CAD build for the part. Positions are in the model's coordinates, mm. A direction names the side the tool comes from. Round coordinates to 2 decimals unless told otherwise and drop trailing zeros. Loops run counter-clockwise (first coordinate to the right, second up) from the corner with the lowest first, then second, coordinate; pieces in that order, holes last. Notation, with made-up numbers: (-35.5, 76.5) - (-0.5, 76.5) arc R21 cw to (-0.5, 113.5) - close; hole circle Ø7 at (24.25, 62.25). An arc over 180 degrees is marked (long way). One line per question, with ' | ' between items.
```python
from build123d import *

# Parameters (mm, degrees)
EXTRUDE_1_DEPTH = 3
EXTRUDE_START   = 6
EXTRUDE_2_DEPTH = 6
EXTRUDE_6_DEPTH = 30
FILLET_1_R      = 1
EXTRUDE_9_DEPTH = 24.000000000000007
FILLET_2_R      = 3


with BuildPart() as part:
    # 草图1 → 凸台-拉伸1 (new body)
    with BuildSketch(Plane(origin=(0, 0, 0), x_dir=(1, 0, 0), z_dir=(0, 1, 0))):
        with BuildLine():
            ThreePointArc((-8.660254037844387, -5.000000000000001), (-2.0048037027267505, -9.796977192661679), (5.999999999999981, -8.000000000000014))
            Line((5.999999999999978, -8), (26.244997998398397, -8))
            Line((26.244997998398397, -8), (26.244997998398397, -5))
            Line((26.244997998398397, -5), (-8.660254037844389, -5))
        make_face()
    extrude(amount=EXTRUDE_1_DEPTH)

    # 草图2 → 凸台-拉伸2 (add)
    with BuildSketch(Plane.XZ.offset(EXTRUDE_START)):
        with BuildLine():
            ThreePointArc((6.000000000000001, 7.999999999999999), (-2.0048037027267367, 9.796977192661682), (-8.660254037844386, 5.0000000000000036))
            Line((-8.660254037844387, 5), (-6.244997998398355, 5))
            ThreePointArc((-6.244997998398368, 5.000000000000037), (7.6e-15, 8), (6.244997998398378, 5.000000000000025))
            Line((6.24499799839837, 5), (8.660254037844625, 5))
            ThreePointArc((8.660254037844535, 4.999999999999743), (7.4820292777785, 6.63469953249319), (6.000000000000001, 7.999999999999999))
        make_face()
    extrude(amount=-EXTRUDE_2_DEPTH)

    # 草图3 → 凸台-拉伸6 (add)
    with BuildSketch(Plane(origin=(0, 0, 5), x_dir=(-1, 0, 0), z_dir=(0, 0, -1))):
        Polygon((-8.660254037844387, 0), (-8.660254037844387, 3.000000000000001), (-11.660254037844386, 3), (-11.660254037844384, 0), align=None)
    extrude(amount=-EXTRUDE_6_DEPTH)

    # 圆角1
    fillet_1_edges = [part.edges().sort_by_distance(p)[0] for p in [
        (7.4820292777784605, 0, 6.634699532493231),
    ]]
    fillet(fillet_1_edges, radius=FILLET_1_R)

    # 草图5 → 凸台-拉伸9 (add)
    with BuildSketch(Plane.XY.offset(34.99999999999999)):
        Polygon((8.660254037844387, -2.0027453895176524), (8.660254037844387, 0), (11.660254037844386, 0), (11.660254037844384, -2.002745389517652), align=None)
    extrude(amount=-EXTRUDE_9_DEPTH)

    # 圆角2
    # the kernel refuses this fillet: 3 mm, written as the material it adds along each edge
    with BuildSketch(Plane(origin=(8.660254037844387, 0, 10.999999999999986), x_dir=(0, -1, 0), z_dir=(1, 0, 0))) as fillet_2_piece_1:
        with BuildLine():
            CenterArc((3, 2.8293962680882476), FILLET_2_R, 180, 70.58438351191461)
            Line((0, 2.8293962680882476), (-0.06, 2.8293962680882476))
            Line((-0.06, 2.8293962680882476), (-0.06, 0))
            Line((-0.06, 0), (0, -0.0600000000000005))
            ThreePointArc((0, -0.0600000000000005), (1.0013726947588264, -0.0600000000000005), (1.9828002973080059, -0.05658792536176449))
            Line((1.9828002973080059, -0.05658792536176449), (2.002745389517653, 0))
        make_face()
    extrude(amount=2.9999999999999982)


solid = part.part
```
(1) Two-plate mould, pull along X, no slides. Class faces 6 (the face through (0, 0, 6)), 7 (the face through (17, 0, 7)), 8 (the face through (11.66, 0, 21)): released by +X, released by -X, zero draft, split by the parting line, or undercut.
Results found:
face 6: undercut | face 7: zero draft | face 8: released by +X
(2) Cut at C-C, the plane y = -3. Write the cut outline in (x, z) (3 decimals).
Results found:
outline: (-8.66, 5) - (-6.245, 5) arc R8 cw to (6.245, 5) - (8.66, 5) arc R10 ccw to start
(3) Cut at D-D, the plane z = 17. Write the cut outline in (x, y), then the cut area to 3 significant figures.
Results found:
outline: (8.66, -2) - (11.66, -2) - (11.66, 3) - (8.66, 3) - close | area: 15.0 mm²
(4) Tool access for faces 1 (the face through (0, -6, 9)), 2 (the face through (0, -3, 8)), 3 (the face through (7, 1, 8)), 4 (the face through (19, 1, 8)), 5 (the face through (10, 1, 35)): list every direction of +Z, -Z, +X, -X, +Y, -Y with a clear straight run to the whole face (end or side of a thin tool).
Results found:
face 1: +Z, -Z, +X, -X, -Y | face 2: -Z, -Y | face 3: +Z, +Y, -Y | face 4: +Z, +X, +Y, -Y | face 5: +Z, +X, -X, +Y, -Y
(5) Drop flat-ended pins along their axis: P1, Ø1.3, axis at x = 7.5, y = 1.5, coming from the +Z side; P2, Ø1.6, axis at x = 20.5, z = 6, coming from the -Y side; P3, Ø1, axis at y = -4, z = 24, coming from the -X side; P4, Ø4, axis at y = 0.5, z = 15, coming from the -X side. Give the stop position or say it passes through.
Results found:
P1: stops at z = 8 | P2: stops at y = 0 | P3: passes through | P4: stops at x = 8.66
(6) Cut at B-B, the plane x = 0. Write the cut outline in (y, z), then the cut area to 3 significant figures.
Results found:
outline: (-6, 8) - (0, 8) - (0, 5) - (3, 5) - (3, 10) - (-6, 10) - close | area: 27.0 mm²
(7) Probe L1, parallel to Z at x = 22.5, y = 0.25; L2, parallel to X at y = -0.25, z = 22; L3, parallel to Z at x = 5, y = -2 (3 decimals). List the from-to ranges inside material, lowest first.
Results found:
L1: z = 5 to 8 | L2: x = 8.66 to 11.66 | L3: z = 6.245 to 8.66
(8) Cut at A-A, the plane z = 9. Write the cut outline in (x, y).
Results found:
outline: (-4.36, -6) - (4.36, -6) - (4.36, 3) - (-4.36, 3) - close; (8.66, -0.12) - (11.66, -0.12) - (11.66, 3) - (8.66, 3) - close
